Autodesk Inventor part; units mm, degrees
ref_plane "YZ Plane" through (0, 0, 0) normal (1, 0, 0) x (0, 1, 0)
ref_plane "XZ Plane" through (0, 0, 0) normal (0, 1, 0) x (-1, 0, 0)
ref_plane "XY Plane" through (0, 0, 0) normal (0, 0, 1) x (1, 0, 0)
sketch "Sketch1" plane through (0, 0, 0) normal (0, 1, 0) x (-1, 0, 0)
  line L0 (0, 0) -> (30, 0)
  line L1 (30, 0) -> (30, -32)
  line L2 (30, -32) -> (0, -32)
  line L3 (0, -32) -> (0, 0)
  dimension "d0" = 30
  dimension "d1" = 32
extrude "Extrusion1" add sketch "Sketch1" along normal blind 15
sketch "Sketch2" plane through (-30, 0, 0) normal (0, 0, 1) x (1, 0, 0)
  line L0 (30, 15) -> (0, 15)
  line L1 (0, 15) -> (30, 0) construction
  line L2 (30, 0) -> (0, 0)
  line L3 (0, 0) -> (30, 15) construction
  circle A0 centre (15, 7.5) radius 3
  dimension "d4" = 6
extrude "Extrusion2" cut sketch "Sketch2" against normal through all
sketch "Sketch3" plane through (0, 15, 0) normal (0, 1, 0) x (1, 0, 0)
  circle A0 centre (-25, 6) radius 1.5
  circle A1 centre (-25, 26) radius 1.5
  circle A2 centre (-5, 6) radius 1.5
  circle A3 centre (-5, 26) radius 1.5
  line L0 (-30, 0) -> (0, 0)
  line L1 (-30, 32) -> (-30, 0)
  line L2 (-5, 26) -> (0, 26) construction
  line L3 (0, 0) -> (0, 32)
  line L4 (-25, 26) -> (-30, 26) construction
  dimension "d7" = 3
  dimension "d8" = 6
  dimension "d9" = 20
  dimension "d10" = 20
extrude "Extrusion3" cut sketch "Sketch3" against normal blind 10
properties part number "AE_MOVING_STAGE"
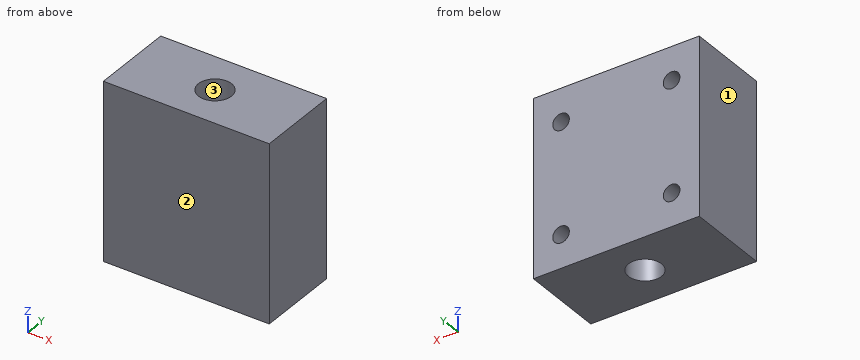
Model file for the job. Use its own axes, mm. Face numbers are marked on the shaded views. Coordinates: 2 decimals unless noted, no trailing zeros. Order: outer loops, then holes, each group sorted by start corner. A loop starts at its lowest first (then second) coordinate and runs counter-clockwise, first axis right, second up. Notation, with made-up numbers: M 16.25,88 L 31.25,88 A7 ccw 31.25,97 Z; hole C 56.5,42.5 d6. An arc over 180 degrees is marked long. Answer as CSV lines item,"result".
(1) Band-saw the part on B-B, the plane x = -15. List the corners of the cut face in (y, z), then the cut area to 3 significant figures.
Geometry says:
outline,"M 0,-32 L 4.5,-32 L 4.5,0 L 0,0 Z; M 10.5,-32 L 15,-32 L 15,0 L 10.5,0 Z"
area,"288 mm2"
(2) Flat gauge pin, fed straight in: pin 1 (0.9 mm diameter, centred on x = -25, z = -26.5, fed in from +Y). Where does the tip first touch, or does it go through?
Geometry says:
pin 1,"stops at y = 5"
(3) Band-saw the part on C-C, the plane z = -6. List the corners of the cut face in (x, y), then the cut area to 3 significant figures.
Geometry says:
outline,"M -30,0 L 0,0 L 0,15 L -3.5,15 L -3.5,5 L -6.5,5 L -6.5,15 L -23.5,15 L -23.5,5 L -26.5,5 L -26.5,15 L -30,15 Z; hole C -15,7.5 d6"
area,"362 mm2"
(4) Wall check: line 1 along Z through (x, y) = (-5, 9.75); line 2 along X through (y, z) = (12, -26); line 3 along X through (y, z) = (10, -6). Give the ranges that are in metal, low to high.
Geometry says:
line 1,"z = -32 to -27.5, -24.5 to -7.5, -4.5 to 0"
line 2,"x = -30 to -26.5, -23.5 to -6.5, -3.5 to 0"
line 3,"x = -30 to -26.5, -23.5 to -16.66, -13.34 to -6.5, -3.5 to 0"
(5) Pull direction Y, two halves, no side cores. Call the marked faces 1, 2 and 3: +Y half, -Y half, draft (parallel to the pull), parting line (faces both ways), or undercut.
Geometry says:
face 1,"draft"
face 2,"-Y half"
face 3,"undercut"
(6) Band-saw the part on A-A, the plane y = 7.5. List the corners of the cut face in (x, z), then the cut area to 3 significant figures.
Geometry says:
outline,"M -30,-32 L -18,-32 L -18,0 L -30,0 Z; M -12,-32 L 0,-32 L 0,0 L -12,0 Z; hole C -25,-26 d3; hole C -25,-6 d3; hole C -5,-26 d3; hole C -5,-6 d3"
area,"740 mm2"
(7) Band-saw the part on D-D, the plane x = -5. List the corners of the cut face in (y, z), then the cut area to 3 significant figures.
Geometry says:
outline,"M 0,-32 L 15,-32 L 15,-27.5 L 5,-27.5 L 5,-24.5 L 15,-24.5 L 15,-7.5 L 5,-7.5 L 5,-4.5 L 15,-4.5 L 15,0 L 0,0 Z"
area,"420 mm2"
